from build123d import *

# Parameters (mm, degrees)
BOSS_EXTRUDE1_DEPTH = 70
SKETCH2_R           = 20
CUT_EXTRUDE1_DEPTH  = 129


with BuildPart() as part:
    # Sketch1 → Boss-Extrude1 (new body)
    with BuildSketch(Plane.XY):
        with BuildLine():
            Line((-187.20703125, 37.086522646), (-187.20703125, -258.837890625))
            Line((-187.20703125, -258.837890625), (-87.20703125, -258.837890625))
            Line((-87.20703125, -258.837890625), (-87.20703125, -68.837890625))
            ThreePointArc((-87.20703125, -68.837890625), (-84.278099062, -61.766822813), (-77.20703125, -58.837890625))
            Line((-77.20703125, -58.837890625), (52.79296875, -58.837890625))
            ThreePointArc((52.79296875, -58.837890625), (59.864036562, -55.908958437), (62.79296875, -48.837890625))
            Line((62.79296875, -48.837890625), (62.79296875, 181.162109375))
            ThreePointArc((62.79296875, 181.162109375), (59.864036562, 188.233177187), (52.79296875, 191.162109375))
            Line((52.79296875, 191.162109375), (-36.375896467, 191.162109375))
            ThreePointArc((-36.375896467, 191.162109375), (-40.255270839, 190.378966458), (-43.527024298, 188.152200272))
            Line((-43.527024298, 188.152200272), (-184.35815908, 44.076613543))
            ThreePointArc((-184.35815908, 44.076613543), (-186.467465319, 40.860692866), (-187.20703125, 37.086522646))
        make_face()
    extrude(amount=BOSS_EXTRUDE1_DEPTH)

    # Sketch2 → Cut-Extrude1 (cut)
    with BuildSketch(Plane(origin=(-87.20703125, 0, 0), x_dir=(0, 0, -1), z_dir=(1, 0, 0))):
        with Locations((-35, -108.837890625)):
            Circle(SKETCH2_R)
        with Locations((-35, -198.837890625)):
            Circle(SKETCH2_R)
    extrude(amount=-CUT_EXTRUDE1_DEPTH, mode=Mode.SUBTRACT)


solid = part.part
Work out the finished part from the listing and answer in its coordinate system (mm). A direction names the side the tool comes from. Give positions to 0.01 mm unless a question says otherwise; leave off trailing zeros. Loops run counter-clockwise (first coordinate to the right, second up) from the corner with the lowest first, then second, coordinate; pieces in that order, holes last. Notation, with made-up numbers: (-12, -2) -> (19, -2) arc R18 ccw to (19, 30) -> close; hole circle Ø6 at (86.5, 67). An arc over 180 degrees is marked (long way). Use a Markdown table: item, result. Add a question column.
1) The part is cut by section B-B, the plane z = 6. Determine the outline of the cut face in (x, y), plus the area to 3 significant figures.
2) For a pull along Z with two mould halves and no side action, classify faces 3 (the cylindrical face through (-84.355, -61.845, 34.51)), 4 (the cylindrical face through (-136.507, -181.974, 24.248)), 5 (the flat face through (-64, -31, 0)), 6 (the cylindrical face through (-136.51, -126.58, 25.77)) as +Z half, -Z half, draft (parallel to the pull), parting line (faces both ways), or undercut.
3) The part is cut by section A-A, the plane z = 35. Determine the outline of the cut face in (x, y), plus the area to 3 significant figures.
4) The part is cut by section C-C, the plane y = -192.5. Determine the outline of the cut face in (x, z), plus the area to 3 significant figures.
5) Consider line 1 along Y through (x, z) = (-164, 35); line 2 along Y through (x, z) = (-123.5, 35); line 3 along Y through (x, z) = (-31, 38). Determine where each line is inside the solid, lowest interval first.
6) The part is cut by section D-D, the plane x = -143. Determine the outline of the cut face in (y, z), plus the area to 3 significant figures.
7) Which of the six approach directions +Z, -Z, +X, -X, +Y, -Y give full straight-line access (tool end or side, diameter ignored) to faces 1 (the flat face through (-187.207, -109, 58)), 2 (the flat face through (-87.207, -165, 35))?
8) Each of these flat-tipped pins is pushed along its axis until it touches: P1, Ø6, axis at x = -157, z = 63, coming from the +Y side; P2, Ø10, axis at y = -145, z = 28.5, coming from the +X side; P3, Ø8, axis at x = -161.5, z = 52.5, coming from the +Y side; P4, Ø24, axis at y = -108.84, z = 35, coming from the -X side. Where does it stop, or does it pass through?
Reported:
| question | item | result |
|---|---|---|
| 1 | outline | (-187.21, -258.84) -> (-87.21, -258.84) -> (-87.21, -68.84) arc R10 cw to (-77.21, -58.84) -> (52.79, -58.84) arc R10 ccw to (62.79, -48.84) -> (62.79, 181.16) arc R10 ccw to (52.79, 191.16) -> (-36.38, 191.16) arc R10 ccw to (-43.53, 188.15) -> (-184.36, 44.08) arc R10 ccw to (-187.21, 37.09) -> close |
| 1 | area | 71,500 mm^2 |
| 2 | face 3 | draft |
| 2 | face 4 | undercut |
| 2 | face 5 | -Z half |
| 2 | face 6 | undercut |
| 3 | outline | (-187.21, -258.84) -> (-87.21, -258.84) -> (-87.21, -218.84) -> (-187.21, -218.84) -> close; (-187.21, -178.84) -> (-87.21, -178.84) -> (-87.21, -128.84) -> (-187.21, -128.84) -> close; (-187.21, -88.84) -> (-87.21, -88.84) -> (-87.21, -68.84) arc R10 cw to (-77.21, -58.84) -> (52.79, -58.84) arc R10 ccw to (62.79, -48.84) -> (62.79, 181.16) arc R10 ccw to (52.79, 191.16) -> (-36.38, 191.16) arc R10 ccw to (-43.53, 188.15) -> (-184.36, 44.08) arc R10 ccw to (-187.21, 37.09) -> close |
| 3 | area | 63,500 mm^2 |
| 4 | outline | (-187.21, 0) -> (-87.21, 0) -> (-87.21, 16.03) -> (-187.21, 16.03) -> close; (-187.21, 53.97) -> (-87.21, 53.97) -> (-87.21, 70) -> (-187.21, 70) -> close |
| 4 | area | 3,210 mm^2 |
| 5 | line 1 | y = -258.84 to -218.84, -178.84 to -128.84, -88.84 to 64.9 |
| 5 | line 2 | y = -258.84 to -218.84, -178.84 to -128.84, -88.84 to 106.34 |
| 5 | line 3 | y = -58.84 to 191.16 |
| 6 | outline | (-258.84, 0) -> (86.39, 0) -> (86.39, 70) -> (-258.84, 70) -> close; hole circle Ø40 at (-198.84, 35); hole circle Ø40 at (-108.84, 35) |
| 6 | area | 21,700 mm^2 |
| 7 | face 1 | +Z, -Z, -X, +Y, -Y |
| 7 | face 2 | +Z, -Z, +X, -Y |
| 8 | P1 | stops at y = 75.13 |
| 8 | P2 | stops at x = -87.21 |
| 8 | P3 | stops at y = 71.55 |
| 8 | P4 | passes through |
